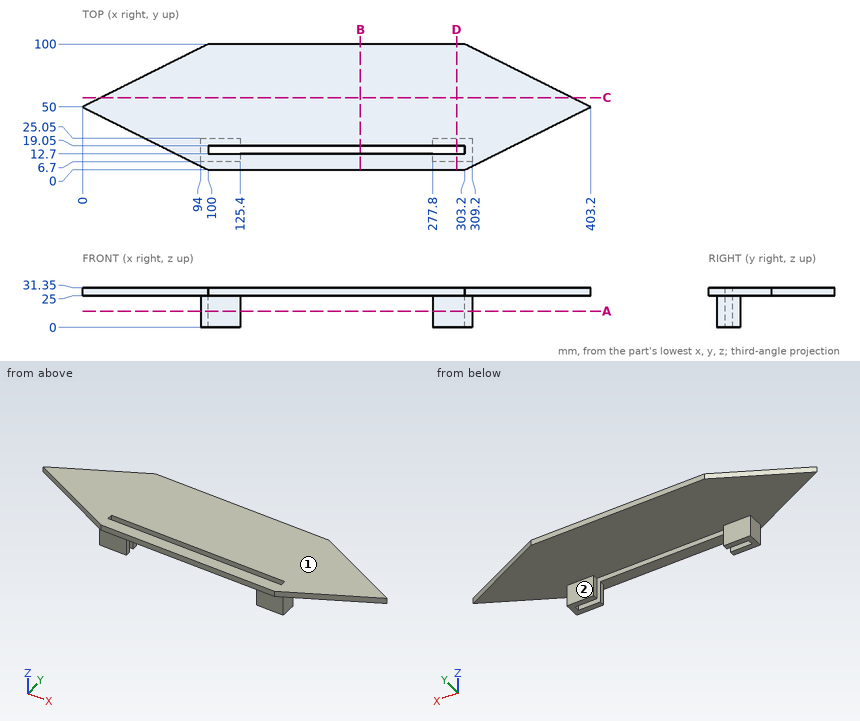
Job drawing, mm, ordinate dimensions from the low corner. One solid piece. A direction names the side the tool comes from. Coordinates: 2 decimals unless noted, no trailing zeros. Order: outer loops, then holes, each group sorted by start corner. A loop starts at its lowest first (then second) coordinate and runs counter-clockwise, first axis right, second up. Notation, with made-up numbers: (-25, 37) - (-18, 37) arc R18 ccw to (-18, 51) - close; hole circle Ø2 at (25, 25). An arc over 180 degrees is marked (long way). Return JSON: item names as keys, results as strings. Group by question number.
1) Saw through at D-D, the plane x = 297. Write the cut outline in (y, z).
2) Saw through at B-B, the plane x = 220.5. Write the cut outline in (y, z), plus the area to 3 significant figures.
3) Saw through at A-A, the plane z = 13. Write the cut outline in (x, y), plus the area to 3 significant figures.
4) Tool access for the marked faces 1 and 2: list every direction of +Z, -Z, +X, -X, +Y, -Y with a clear straight run to the whole face (end or side of a thin tool).
5) Saw through at C-C, the plane y = 57.5. Write the cut outline in (x, z).
6) Flat gauge pins, fed straight in: P1, Ø1.8, axis at y = 9, z = 6.5, coming from the +X side; P2, Ø8, axis at x = 266, y = 76.5, coming from the -Z side; P3, Ø5, axis at y = 14.5, z = 8.5, coming from the -X side. Where does each tip first touch, or does it go through?
7) Probe line 1 (Y direction, x = 234, z = 30); line 2 (Y direction, x = 282.5, z = 24); line 3 (Z direction, x = 125.5, y = 65). List the from-to ranges inside material, lowest first. Write a range as from..to.
Values found:
{
 "1": {"outline": "(0, 25) - (6.7, 25) - (6.7, 0) - (12.7, 0) - (12.7, 31.35) - (0, 31.35) - close; (19.05, 0) - (25.05, 0) - (25.05, 25) - (100, 25) - (100, 31.35) - (19.05, 31.35) - close"},
 "2": {"outline": "(0, 25) - (12.7, 25) - (12.7, 31.35) - (0, 31.35) - close; (19.05, 25) - (100, 25) - (100, 31.35) - (19.05, 31.35) - close", "area": "595 mm²"},
 "3": {"outline": "(94, 6.7) - (125.4, 6.7) - (125.4, 12.7) - (100, 12.7) - (100, 19.05) - (125.4, 19.05) - (125.4, 25.05) - (94, 25.05) - close; (277.8, 6.7) - (309.2, 6.7) - (309.2, 25.05) - (277.8, 25.05) - (277.8, 19.05) - (303.2, 19.05) - (303.2, 12.7) - (277.8, 12.7) - close", "area": "830 mm²"},
 "4": {"face 1": "+Z, +X, -X, +Y, -Y", "face 2": "-Z, +X, -X, +Y"},
 "5": {"outline": "(15, 25) - (388.2, 25) - (388.2, 31.35) - (15, 31.35) - close"},
 "6": {"P1": "stops at x = 309.2", "P2": "stops at z = 25", "P3": "stops at x = 94"},
 "7": {"line 1": "y = 0..12.7, 19.05..100", "line 2": "y = 6.7..12.7, 19.05..25.05", "line 3": "z = 25..31.35"}
}
